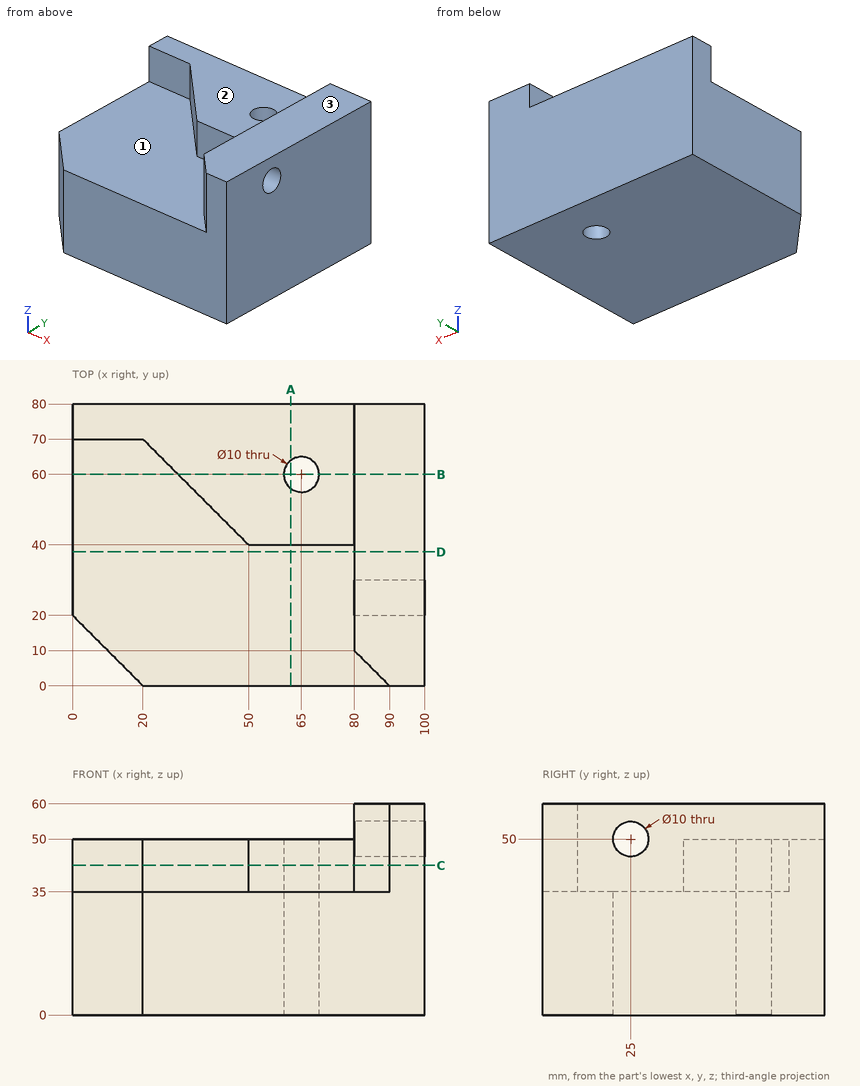
Print and shaded views of the part. All mm, measured from the part's lowest x, y and z. A direction names the side the tool comes from. Coordinates: 2 decimals unless noted, no trailing zeros. Loops run counter-clockwise (first coordinate to the right, second up) from the corner with the lowest first, then second, coordinate; pieces in that order, holes last. Notation, with made-up numbers: M -2.5,-32 L 7.5,-32 A12 ccw 7.5,-25 Z; hole C 50,-12 d1. An arc over 180 degrees is marked long. Use a Markdown table: item, result. Add a question column.
Q1. Pin check, flat tips, straight feed: P1, Ø20, axis at x = 50, y = 58.5, coming from the +Z side; P2, Ø3, axis at x = 60, z = 25, coming from the -Y side; P3, Ø7.5, axis at y = 42, z = 51, coming from the -X side; P4, Ø12, axis at x = 70.5, z = 44.5, coming from the -Y side. Stop position of each tip, or through.
Q2. Cut at C-C (z = 42.5). Write the cut outline in (x, y), and give its area (3 significant figures).
Q3. Cut at D-D (y = 38). Write the cut outline in (x, z), and give its area (3 significant figures).
Q4. Probe L1, parallel to Z at x = 90.75, y = 25; L2, parallel to X at y = 60, z = 28.5; L3, parallel to X at y = 60, z = 36. List the from-to ranges inside material, lowest first.
Q5. Which spindle directions (+Z, -Z, +X, -X, +Y, -Y) get a long thin tool onto all of the face, cutting with end or side? Do the marked faces 1, 2 and 3. Say none if no direction does.
Q6. Cut at A-A (x = 62). Write the cut outline in (y, z), and give its area (3 significant figures).
Q7. Cut at B-B (y = 60). Write the cut outline in (x, z).
Worked out:
| question | item | result |
|---|---|---|
| 1 | P1 | stops at z = 50 |
| 1 | P2 | stops at y = 0 |
| 1 | P3 | stops at x = 44.39 |
| 1 | P4 | stops at y = 40 |
| 2 | outline | M 0,70 L 20,70 L 50,40 L 80,40 L 80,10 L 90,0 L 100,0 L 100,80 L 0,80 Z; hole C 65,60 d10 |
| 2 | area | 3,620 mm2 |
| 3 | outline | M 0,0 L 100,0 L 100,60 L 80,60 L 80,35 L 0,35 Z |
| 3 | area | 4,000 mm2 |
| 4 | L1 | z = 0 to 45, 55 to 60 |
| 4 | L2 | x = 0 to 60, 70 to 100 |
| 4 | L3 | x = 30 to 60, 70 to 100 |
| 5 | face 1 | +Z, -X, -Y |
| 5 | face 2 | +Z, -X, +Y, -Y |
| 5 | face 3 | +Z, +X, -X, +Y, -Y |
| 6 | outline | M 0,0 L 56,0 L 56,50 L 40,50 L 40,35 L 0,35 Z; M 64,0 L 80,0 L 80,50 L 64,50 Z |
| 6 | area | 3,000 mm2 |
| 7 | outline | M 0,0 L 60,0 L 60,50 L 30,50 L 30,35 L 0,35 Z; M 70,0 L 100,0 L 100,60 L 80,60 L 80,50 L 70,50 Z |
